The figure shows three views and two pictorial views of one solid part (mm, origin at its lowest corner). Answer the questions. A direction names the side the tool comes from. Give positions to 0.01 mm unless a question says otherwise; leave off trailing zeros. Write each loop counter-clockwise with the first axis right and the second up, starting at its lowest first coordinate (ties: lowest second). Pieces come first, ordered by that corner, then holes. Notation, with made-up numbers: (27, 19) -> (64, 19) arc R22 cw to (64, 52) -> close; hole circle Ø10 at (64.5, -15). An arc over 180 degrees is marked (long way). Use a Markdown table: item, result.
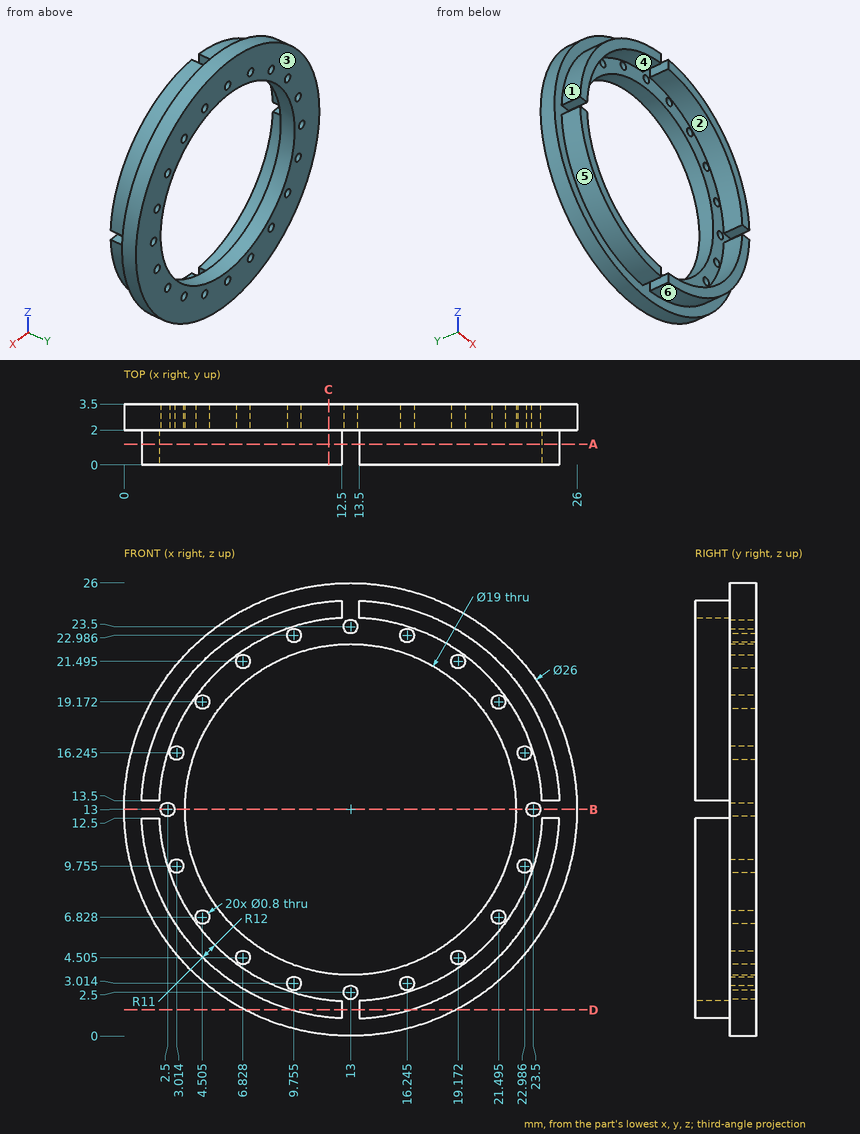
Item 1: A cutting plane is placed at B-B (z = 13). Give the vertices of the cut face in (x, y).
Return value:
| item | result |
|---|---|
| outline | (0, 2) -> (2.1, 2) -> (2.1, 3.5) -> (0, 3.5) -> close; (2.9, 2) -> (3.5, 2) -> (3.5, 3.5) -> (2.9, 3.5) -> close; (22.5, 2) -> (23.1, 2) -> (23.1, 3.5) -> (22.5, 3.5) -> close; (23.9, 2) -> (26, 2) -> (26, 3.5) -> (23.9, 3.5) -> close |
Item 2: A cutting plane is placed at D-D (z = 1.5). Give the vertices of the cut face in (x, y), then the cut area to 3 significant figures.
Return value:
| item | result |
|---|---|
| outline | (6.94, 2) -> (9.57, 2) -> (9.57, 0) -> (12.5, 0) -> (12.5, 2) -> (13.5, 2) -> (13.5, 0) -> (16.43, 0) -> (16.43, 2) -> (19.06, 2) -> (19.06, 3.5) -> (6.94, 3.5) -> close |
| area | 29.9 mm^2 |
Item 3: A cutting plane is placed at C-C (x = 11.75). Give the vertices of the cut face in (y, z) (1 decimal).
Return value:
| item | result |
|---|---|
| outline | (0, 1.1) -> (2, 1.1) -> (2, 0.1) -> (3.5, 0.1) -> (3.5, 3.6) -> (2, 3.6) -> (2, 2.1) -> (0, 2.1) -> close; (0, 23.9) -> (2, 23.9) -> (2, 22.4) -> (3.5, 22.4) -> (3.5, 25.9) -> (2, 25.9) -> (2, 24.9) -> (0, 24.9) -> close |
Item 4: A cutting plane is placed at A-A (y = 1.2). Give the vertices of the cut face in (x, z).
Return value:
| item | result |
|---|---|
| outline | (1.01, 12.5) arc R12 ccw to (12.5, 1.01) -> (12.5, 2.01) arc R11 cw to (2.01, 12.5) -> close; (1.01, 13.5) -> (2.01, 13.5) arc R11 cw to (12.5, 23.99) -> (12.5, 24.99) arc R12 ccw to start; (13.5, 1.01) arc R12 ccw to (24.99, 12.5) -> (23.99, 12.5) arc R11 cw to (13.5, 2.01) -> close; (13.5, 23.99) arc R11 cw to (23.99, 13.5) -> (24.99, 13.5) arc R12 ccw to (13.5, 24.99) -> close |
Item 5: Straight lines are drawn through the part: line 1 along X through (y, z) = (2.55, 13); line 2 along Z through (x, y) = (9.5, 3.2) (1 decimal); line 3 along Z through (x, y) = (21.75, 2.3) (1 decimal). For each, find the intervals that lie inside material, in ascending order. Write a range as [from, to].
Return value:
| item | result |
|---|---|
| line 1 | [0, 2.1], [2.9, 3.5], [22.5, 23.1], [23.9, 26] |
| line 2 | [0.5, 2.7], [3.3, 4.2], [21.8, 22.7], [23.3, 25.5] |
| line 3 | [3.4, 6.5], [7.1, 9.3], [16.7, 18.9], [19.5, 22.6] |
Item 6: A tool of negligible diameter and unlimited length cuts with its end or side. For the marked faces 1, 2 and 3, from which of +Z, -Z, +X, -X, +Y, -Y can it reach the whole face along a straight path? Write none if from no direction.
Return value:
| item | result |
|---|---|
| face 1 | +Z, -X, -Y |
| face 2 | -Y |
| face 3 | +Z, -Z, +X, -X, +Y |
Item 7: For a pull along X with two mould halves and no side action, classify the marked faces 4, 5 and 6 as +X half, -X half, draft (parallel to the pull), parting line (faces both ways), or undercut.
Return value:
| item | result |
|---|---|
| face 4 | undercut |
| face 5 | -X half |
| face 6 | +X half |
Item 8: Each of these flat-tipped pins is pushed along its axis until it touches: P1, Ø1.1, axis at x = 24.5, y = 0.5, coming from the -Z side; P2, Ø1, axis at y = 3, z = 9.5, coming from the +X side; P3, Ø0.8, axis at x = 24.5, y = 1, coming from the +Z side. Where does it stop, or does it pass through?
Return value:
| item | result |
|---|---|
| P1 | z = 8.09 |
| P2 | x = 25.65 |
| P3 | z = 17.56 |
